Design review of the part built by this model. Coordinates are the model's own, in mm. A direction names the side the tool comes from. Give positions to 0.01 mm unless a question says otherwise; leave off trailing zeros. Order: outer loops, then holes, each group sorted by start corner. A loop starts at its lowest first (then second) coordinate and runs counter-clockwise, first axis right, second up. Notation, with made-up numbers: M 0,67 L 4,67 A8 cw 4,77 Z; hole C -13.5,-15.75 d9. An arc over 180 degrees is marked long. Put each result on its own line as item: value. Start each with the question number.
from build123d import *

# Parameters (mm, degrees)
SKETCH_1_W          = 155
SKETCH_1_H          = 60.5
SKETCH_1_R          = 13.5
SKETCH_1_R_2        = 1.55
EXTRUDE_1_DEPTH     = 5
SKETCH_3_W          = 30
SKETCH_3_H          = 40
EXTRUDE_2_DEPTH     = 5
SKETCH_4_W          = 155
SKETCH_4_H          = 10
EXTRUDE_3_DEPTH     = 5
CUT_EXTRUDE_1_DEPTH = 104.885754558
SKETCH_6_R          = 2.1
CUT_EXTRUDE_2_DEPTH = 104.885754558
SKETCH_7_R          = 1.55
SKETCH_7_R_2        = 2.05
CUT_EXTRUDE_3_DEPTH = 104.885754558
EXTRUDE_6_DEPTH     = 5
CUT_EXTRUDE_4_DEPTH = 5
SKETCH_13_R         = 1.55
CUT_EXTRUDE_5_DEPTH = 104.885754558
FILLET_1_R          = 1
FILLET_2_R          = 2
EXTRUDE_8_DEPTH     = 5
FILLET_3_R          = 2
FILLET_4_R          = 3
SKETCH_15_R         = 1.55
SKETCH_15_R_2       = 1.6
EXTRUDE_9_DEPTH     = 5
FILLET_5_R          = 5
FILLET_6_R          = 8
SKETCH_16_R         = 1.6
CUT_EXTRUDE_6_DEPTH = 110.786201319


with BuildPart() as part:
    # 草图1 → 凸台-拉伸1 (new body)
    with BuildSketch(Plane(origin=(0, 0, 0), x_dir=(1, 0, 0), z_dir=(0, 1, 0))):
        with Locations((0, 1.25)):
            Rectangle(SKETCH_1_W, SKETCH_1_H)
        with Locations(Location((36.5, 0, 0), (0, 0, 270))):
            Circle(SKETCH_1_R, mode=Mode.SUBTRACT)
        with Locations(Location((-36.5, 0, 0), (0, 0, 270))):
            Circle(SKETCH_1_R, mode=Mode.SUBTRACT)
        with Locations(Location((36.5, 17.5, 0), (0, 0, 270))):
            Circle(SKETCH_1_R_2, mode=Mode.SUBTRACT)
        with Locations(Location((45.25, 15.155444566, 0), (0, 0, 270))):
            Circle(SKETCH_1_R_2, mode=Mode.SUBTRACT)
        with Locations(Location((51.655444566, 8.75, 0), (0, 0, 270))):
            Circle(SKETCH_1_R_2, mode=Mode.SUBTRACT)
        with Locations(Location((54, 0, 0), (0, 0, 270))):
            Circle(SKETCH_1_R_2, mode=Mode.SUBTRACT)
        with Locations(Location((51.655444566, -8.75, 0), (0, 0, 270))):
            Circle(SKETCH_1_R_2, mode=Mode.SUBTRACT)
        with Locations(Location((45.25, -15.155444566, 0), (0, 0, 270))):
            Circle(SKETCH_1_R_2, mode=Mode.SUBTRACT)
        with Locations(Location((36.5, -17.5, 0), (0, 0, 270))):
            Circle(SKETCH_1_R_2, mode=Mode.SUBTRACT)
        with Locations(Location((27.75, -15.155444566, 0), (0, 0, 270))):
            Circle(SKETCH_1_R_2, mode=Mode.SUBTRACT)
        with Locations(Location((21.344555434, -8.75, 0), (0, 0, 270))):
            Circle(SKETCH_1_R_2, mode=Mode.SUBTRACT)
        with Locations(Location((19, 0, 0), (0, 0, 270))):
            Circle(SKETCH_1_R_2, mode=Mode.SUBTRACT)
        with Locations(Location((21.344555434, 8.75, 0), (0, 0, 270))):
            Circle(SKETCH_1_R_2, mode=Mode.SUBTRACT)
        with Locations(Location((27.75, 15.155444566, 0), (0, 0, 270))):
            Circle(SKETCH_1_R_2, mode=Mode.SUBTRACT)
        with Locations(Location((-36.5, 17.5, 0), (0, 0, 90))):
            Circle(SKETCH_1_R_2, mode=Mode.SUBTRACT)
        with Locations(Location((-27.75, 15.155444566, 0), (0, 0, 90))):
            Circle(SKETCH_1_R_2, mode=Mode.SUBTRACT)
        with Locations(Location((-21.344555434, 8.75, 0), (0, 0, 90))):
            Circle(SKETCH_1_R_2, mode=Mode.SUBTRACT)
        with Locations(Location((-19, 0, 0), (0, 0, 90))):
            Circle(SKETCH_1_R_2, mode=Mode.SUBTRACT)
        with Locations(Location((-21.344555434, -8.75, 0), (0, 0, 90))):
            Circle(SKETCH_1_R_2, mode=Mode.SUBTRACT)
        with Locations(Location((-27.75, -15.155444566, 0), (0, 0, 90))):
            Circle(SKETCH_1_R_2, mode=Mode.SUBTRACT)
        with Locations(Location((-36.5, -17.5, 0), (0, 0, 90))):
            Circle(SKETCH_1_R_2, mode=Mode.SUBTRACT)
        with Locations(Location((-45.25, -15.155444566, 0), (0, 0, 90))):
            Circle(SKETCH_1_R_2, mode=Mode.SUBTRACT)
        with Locations(Location((-51.655444566, -8.75, 0), (0, 0, 90))):
            Circle(SKETCH_1_R_2, mode=Mode.SUBTRACT)
        with Locations(Location((-54, 0, 0), (0, 0, 90))):
            Circle(SKETCH_1_R_2, mode=Mode.SUBTRACT)
        with Locations(Location((-51.655444566, 8.75, 0), (0, 0, 90))):
            Circle(SKETCH_1_R_2, mode=Mode.SUBTRACT)
        with Locations(Location((-45.25, 15.155444566, 0), (0, 0, 90))):
            Circle(SKETCH_1_R_2, mode=Mode.SUBTRACT)
    extrude(amount=EXTRUDE_1_DEPTH)

    # 草图3 → 凸台-拉伸2 (add)
    with BuildSketch(Plane(origin=(0, 5, 0), x_dir=(1, 0, 0), z_dir=(0, 1, 0))):
        with Locations((0, -49)):
            Rectangle(SKETCH_3_W, SKETCH_3_H)
    extrude(amount=-EXTRUDE_2_DEPTH)

    # 草图4 → 凸台-拉伸3 (add)
    with BuildSketch(Plane(origin=(0, 5, 0), x_dir=(1, 0, 0), z_dir=(0, 1, 0))):
        with Locations((0, 36.5)):
            Rectangle(SKETCH_4_W, SKETCH_4_H)
    extrude(amount=-EXTRUDE_3_DEPTH)

    # 草图5 → 切除-拉伸1 (cut, through all)
    with BuildSketch(Plane.XZ):
        Polygon((-77.5, 29), (-77.5, -6.5), (-42, 29), align=None)
        Polygon((-34.75, -31.5), (-69.5, -41.5), (0, -41.5), (0, -31.5), align=None)
    cut_extrude_1 = extrude(amount=-CUT_EXTRUDE_1_DEPTH, mode=Mode.SUBTRACT)

    # 镜向1: 切除-拉伸1 across plane
    add(cut_extrude_1.mirror(Plane(origin=(0, 0, 0), x_dir=(0, 0, 1), z_dir=(1, 0, 0))), mode=Mode.SUBTRACT)

    # 草图6 → 切除-拉伸2 (cut, through all)
    with BuildSketch(Plane(origin=(0, 5, 0), x_dir=(1, 0, 0), z_dir=(0, 1, 0))):
        with Locations(Location((-73.5, 36.5, 0), (0, 0, 270))):
            Circle(SKETCH_6_R)
        with Locations(Location((-73.5, 11.5, 0), (0, 0, 270))):
            Circle(SKETCH_6_R)
        with Locations(Location((73.5, 11.5, 0), (0, 0, 90))):
            Circle(SKETCH_6_R)
        with Locations(Location((73.5, 36.5, 0), (0, 0, 90))):
            Circle(SKETCH_6_R)
    extrude(amount=-CUT_EXTRUDE_2_DEPTH, mode=Mode.SUBTRACT)

    # 草图7 → 切除-拉伸3 (cut, through all)
    with BuildSketch(Plane(origin=(0, 5, 0), x_dir=(1, 0, 0), z_dir=(0, 1, 0))):
        with Locations(Location((7.5, 28.5, 0), (0, 0, 270))):
            Circle(SKETCH_7_R)
        with Locations(Location((-7.5, 28.5, 0), (0, 0, 270))):
            Circle(SKETCH_7_R)
        with Locations(Location((11, -25, 0), (0, 0, 270))):
            Circle(SKETCH_7_R_2)
        with Locations(Location((-11, -25, 0), (0, 0, 270))):
            Circle(SKETCH_7_R_2)
    extrude(amount=-CUT_EXTRUDE_3_DEPTH, mode=Mode.SUBTRACT)

    # 草图10 → 凸台-拉伸6 (add)
    with BuildSketch(Plane(origin=(0, 5, 0), x_dir=(1, 0, 0), z_dir=(0, 1, 0))):
        Polygon((-42, -29), (-15, -56), (-15, -29), align=None)
        Polygon((15, -29), (15, -56), (42, -29), align=None)
    extrude(amount=-EXTRUDE_6_DEPTH)

    # 草图11 → 切除-拉伸4 (cut)
    with BuildSketch(Plane(origin=(0, 5, 0), x_dir=(1, 0, 0), z_dir=(0, 1, 0))):
        Polygon((-15, -26), (-37.928932188, -26), (-15, -48.928932188), align=None)
        Polygon((15, -26), (15, -48.928932188), (37.928932188, -26), align=None)
    extrude(amount=-CUT_EXTRUDE_4_DEPTH, mode=Mode.SUBTRACT)

    # 草图13 → 切除-拉伸5 (cut, through all)
    with BuildSketch(Plane(origin=(0, 5, 0), x_dir=(1, 0, 0), z_dir=(0, 1, 0))):
        with BuildLine():
            Line((-10, -63.45), (10, -63.45))
            Line((10, -63.45), (10, -41.85))
            ThreePointArc((10, -41.85), (7.489770927, -40.810229073), (6.45, -38.3))
            Line((6.45, -38.3), (-6.45, -38.3))
            ThreePointArc((-6.45, -38.3), (-7.489770927, -40.810229073), (-10, -41.85))
            Line((-10, -41.85), (-10, -63.45))
        make_face()
        with Locations(Location((10, -67, 0), (0, 0, 270))):
            Circle(SKETCH_13_R)
        with Locations(Location((-10, -67, 0), (0, 0, 270))):
            Circle(SKETCH_13_R)
        with Locations(Location((10, -38.3, 0), (0, 0, 270))):
            Circle(SKETCH_13_R)
        with Locations(Location((-10, -38.3, 0), (0, 0, 270))):
            Circle(SKETCH_13_R)
    extrude(amount=-CUT_EXTRUDE_5_DEPTH, mode=Mode.SUBTRACT)

    # 圆角1
    fillet_1_edges = [part.edges().sort_by_distance(p)[0] for p in [
        (-15, 2.5, 26),
        (-15, 2.5, 48.928932188),
        (-37.928932188, 2.5, 26),
        (15, 2.5, 26),
        (37.928932188, 2.5, 26),
        (15, 2.5, 48.928932188),
        (6.45, 2.5, 38.3),
        (10, 2.5, 41.85),
        (10, 2.5, 63.45),
        (-10, 2.5, 63.45),
        (-10, 2.5, 41.85),
        (-6.45, 2.5, 38.3),
    ]]
    fillet(fillet_1_edges, radius=FILLET_1_R)

    # 圆角2
    fillet_2_edges = [part.edges().sort_by_distance(p)[0] for p in [
        (-15, 2.5, 69),
        (15, 2.5, 69),
        (-77.5, 2.5, -41.5),
        (77.5, 2.5, -41.5),
        (-77.5, 2.5, -6.5),
        (-69.5, 2.5, -41.5),
        (-34.75, 2.5, -31.5),
        (77.5, 2.5, -6.5),
        (34.75, 2.5, -31.5),
        (69.5, 2.5, -41.5),
        (-15, 2.5, 56),
        (15, 2.5, 56),
    ]]
    fillet(fillet_2_edges, radius=FILLET_2_R)

    # 草图14 → 凸台-拉伸8 (add)
    with BuildSketch(Plane(origin=(0, 5, 0), x_dir=(1, 0, 0), z_dir=(0, 1, 0))):
        with BuildLine():
            Line((-19.782046737, 41.5), (-69.782046737, 41.5))
            ThreePointArc((-69.782046737, 41.5), (-69.502763464, 41.480404215), (-69.228952966, 41.422000853))
            Line((-69.228952966, 41.422000853), (-62.55, 39.5))
            Line((-62.55, 39.5), (-21.782046737, 39.5))
            Line((-21.782046737, 39.5), (-21.782046737, 31.5))
            Line((-21.782046737, 31.5), (-19.782046737, 31.5))
            Line((-19.782046737, 31.5), (-19.782046737, 41.5))
        make_face()
    extrude_8 = extrude(amount=-EXTRUDE_8_DEPTH)

    # 镜向2: 凸台-拉伸8 across plane
    add(extrude_8.mirror(Plane(origin=(0, 0, 0), x_dir=(0, 0, 1), z_dir=(1, 0, 0))))

    # 圆角3
    fillet_3_edges = [part.edges().sort_by_distance(p)[0] for p in [
        (-19.782046737, 2.5, -41.5),
        (-21.782046737, 2.5, -31.5),
        (-21.782046737, 2.5, -39.5),
        (-62.55, 2.5, -39.5),
        (62.55, 2.5, -39.5),
        (21.782046737, 2.5, -39.5),
        (21.782046737, 2.5, -31.5),
        (19.782046737, 2.5, -41.5),
    ]]
    fillet(fillet_3_edges, radius=FILLET_3_R)

    # 圆角4
    fillet_4_edges = [part.edges().sort_by_distance(p)[0] for p in [
        (-19.782046737, 2.5, -31.5),
        (19.782046737, 2.5, -31.5),
    ]]
    fillet(fillet_4_edges, radius=FILLET_4_R)

    # 草图15 → 凸台-拉伸9 (add)
    # profile 1 of 2: a face of its own
    with BuildSketch(Plane(origin=(0, 5, 0), x_dir=(1, 0, 0), z_dir=(0, 1, 0))):
        with BuildLine():
            Line((8.594020551, -70.314094415), (25.094020551, -77.314094415))
            ThreePointArc((25.094020551, -77.314094415), (29.814094415, -75.405979449), (27.905979449, -70.685905585))
            Line((27.905979449, -70.685905585), (11.405979449, -63.685905585))
            ThreePointArc((11.405979449, -63.685905585), (6.685905585, -65.594020551), (8.594020551, -70.314094415))
        make_face()
        with Locations(Location((10, -67, 0), (0, 0, 270))):
            Circle(SKETCH_15_R, mode=Mode.SUBTRACT)
        with Locations(Location((26.5, -74, 0), (0, 0, 270))):
            Circle(SKETCH_15_R_2, mode=Mode.SUBTRACT)
    # profile 2 of 2: a face of its own
    with BuildSketch(Plane(origin=(0, 5, 0), x_dir=(1, 0, 0), z_dir=(0, 1, 0))):
        with BuildLine():
            Line((-11.405979449, -63.685905585), (-27.905979449, -70.685905585))
            ThreePointArc((-27.905979449, -70.685905585), (-29.814094415, -75.405979449), (-25.094020551, -77.314094415))
            Line((-25.094020551, -77.314094415), (-8.594020551, -70.314094415))
            ThreePointArc((-8.594020551, -70.314094415), (-6.685905585, -65.594020551), (-11.405979449, -63.685905585))
        make_face()
        with Locations(Location((-10, -67, 0), (0, 0, 270))):
            Circle(SKETCH_15_R, mode=Mode.SUBTRACT)
        with Locations(Location((-26.5, -74, 0), (0, 0, 270))):
            Circle(SKETCH_15_R_2, mode=Mode.SUBTRACT)
    extrude(amount=-EXTRUDE_9_DEPTH)

    # 圆角5
    fillet_5_edges = [part.edges().sort_by_distance(p)[0] for p in [
        (7.006674091, 2.5, 69),
        (-7.006674091, 2.5, 69),
    ]]
    fillet(fillet_5_edges, radius=FILLET_5_R)

    # 圆角6
    fillet_6_edges = [part.edges().sort_by_distance(p)[0] for p in [
        (15, 2.5, 65.210641577),
        (-15, 2.5, 65.210641577),
    ]]
    fillet(fillet_6_edges, radius=FILLET_6_R)

    # 草图16 → 切除-拉伸6 (cut, through all)
    with BuildSketch(Plane(origin=(0, 5, 0), x_dir=(1, 0, 0), z_dir=(0, 1, 0))):
        with Locations(Location((-63.5, 36.5, 0), (0, 0, 270))):
            Circle(SKETCH_16_R)
        with Locations(Location((-63.5, 11.5, 0), (0, 0, 270))):
            Circle(SKETCH_16_R)
        with Locations(Location((63.5, 11.5, 0), (0, 0, 270))):
            Circle(SKETCH_16_R)
        with Locations(Location((63.5, 36.5, 0), (0, 0, 270))):
            Circle(SKETCH_16_R)
    extrude(amount=-CUT_EXTRUDE_6_DEPTH, mode=Mode.SUBTRACT)


solid = part.part
1. Machinability: for faces 1 (the flat face through (23.947, 2.535, 69.006)), 2 (the flat face through (-47, 3, 24)), 3 (the flat face through (21.782, 3, -36)), which of the approach directions +Z, -Z, +X, -X, +Y, -Y give a long, thin tool a straight path to every point of the face, cutting with its end or side? Answer none if there is none.
2. Insertion check: pin 1 (3 mm diameter, centred on x = 34.5, y = 4.5, fed in from +Z); pin 2 (1.9 mm diameter, centred on x = -27.75, z = -15.16, fed in from +Y); pin 3 (2.5 mm diameter, centred on x = 2, y = 1.5, fed in from +Z); pin 4 (4 mm diameter, centred on x = 21.34, z = -8.75, fed in from +Y). Each pin has a flat end and moves straight along its axis. Give the tip position at first contact, or say it passes through.
3. Consider section B-B on x = -67. Give the boundary of the cut face in (y, z), then the cut area to 4 significant figures.
4. The part is to be moulded in two halves that separate along Z. For faces 4 (the flat face through (-19.782, 3, -37)), 5 (the cylindrical face through (18.927, 2.465, -32.402)), 6 (the cylindrical face through (-74.778, 2.535, -13.166)), say which applies: +Z half, -Z half, draft (parallel to the pull), parting line (faces both ways), or undercut.
5. Consider section C-C on y = 3.05. Give the number of separate pieces and of enclosed holes in the cut face, then the cut area to 3 significant figures.
6. To check wall thickness, follow probe 1 along X at (y, z) = (2.2, -17.5); probe 2 along Z at (x, y) = (0.5, 4.45); probe 3 along X at (y, z) = (1.05, -14.5). State the ranges of each line that lie inside material, in increasing order.
7. Consider section A-A on x = 2.5. Give the boundary of the cut face in (y, z), then the cut area to 3 significant figures.
Returned:
1. face 1: +X, +Y, -Y
1. face 2: -X, +Y, -Y
1. face 3: +Y, -Y
2. pin 1: stops at z = 38
2. pin 2: passes through
2. pin 3: stops at z = 69
2. pin 4: stops at y = 5
3. outline: M 0,-41.5 L 5,-41.5 L 5,4 L 0,4 Z
3. area: 227.5 mm2
4. face 4: draft
4. face 5: -Z half
4. face 6: undercut
5. separate pieces: 1
5. enclosed holes: 49
5. area: 8,580 mm2
6. probe 1: x = -77.5 to -38.05, -34.95 to 34.95, 38.05 to 77.5
6. probe 2: z = -31.5 to 38.3, 63.45 to 69
6. probe 3: x = -77.5 to -46.65, -43.85 to -29.15, -26.35 to 26.35, 29.15 to 43.85, 46.65 to 77.5
7. outline: M 0,-31.5 L 5,-31.5 L 5,38.3 L 0,38.3 Z; M 0,63.45 L 5,63.45 L 5,69 L 0,69 Z
7. area: 377 mm2
